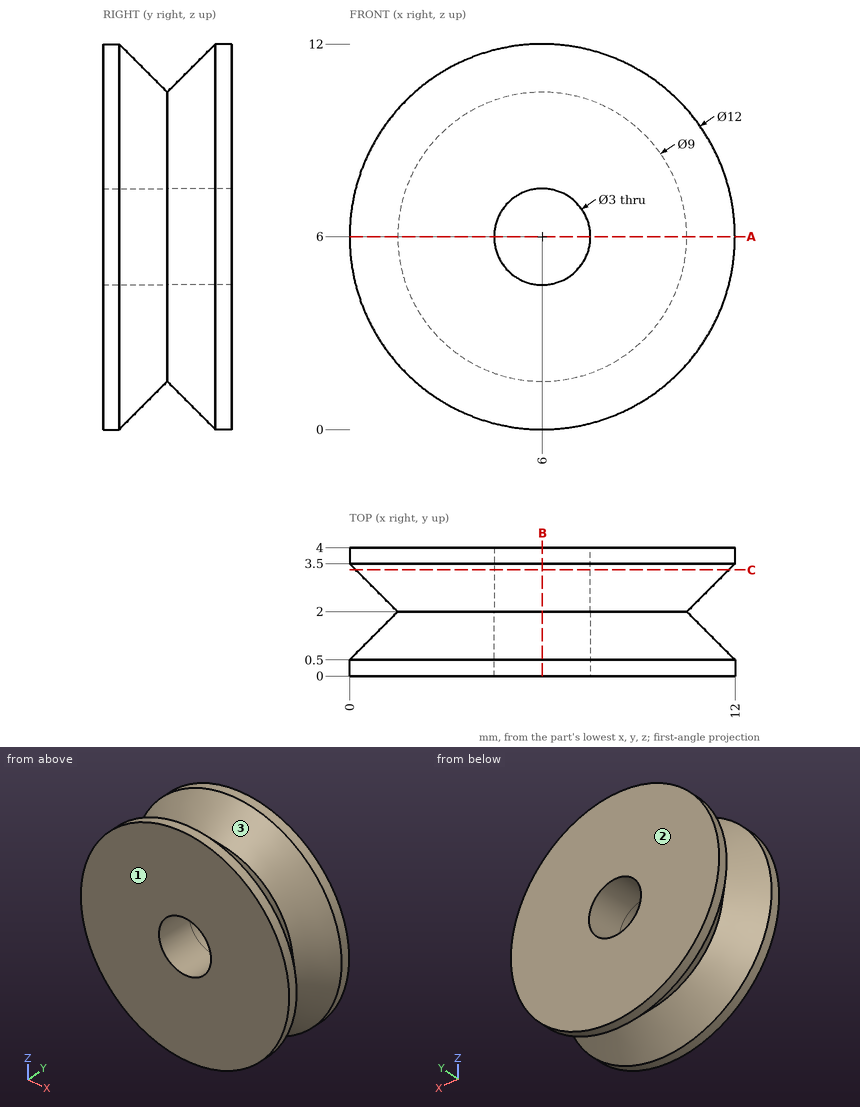
Part print with two shaded views. Sizes in mm from the minimum x, y, z corner. Give positions to 0.01 mm unless a question says otherwise; leave off trailing zeros. Order: outer loops, then holes, each group sorted by start corner. A loop starts at its lowest first (then second) coordinate and runs counter-clockwise, first axis right, second up. Notation, with made-up numbers: M 70.25,55.5 L 89.25,55.5 A14 ccw 89.25,67.5 Z; hole C 14.25,36 d11. An arc over 180 degrees is marked long. Put each result on its own line as item: value.
Item 1: Cut at C-C on y = 3.3. Write the cut outline in (x, z).
Results are:
outline: C 6,6 d11.6; hole C 6,6 d3
Item 2: Cut at A-A on z = 6. Write the cut outline in (x, y).
Results are:
outline: M 0,0 L 4.5,0 L 4.5,4 L 0,4 L 0,3.5 L 1.5,2 L 0,0.5 Z; M 7.5,0 L 12,0 L 12,0.5 L 10.5,2 L 12,3.5 L 12,4 L 7.5,4 Z
Item 3: Pull direction Y, two halves, no side cores. Call the marked faces 1, 2 and 3: +Y half, -Y half, draft (parallel to the pull), parting line (faces both ways), or undercut.
Results are:
face 1: -Y half
face 2: +Y half
face 3: undercut
Item 4: Cut at B-B on x = 6. Write the cut outline in (y, z), then the cut area to 3 significant figures.
Results are:
outline: M 0,0 L 0.5,0 L 2,1.5 L 3.5,0 L 4,0 L 4,4.5 L 0,4.5 Z; M 0,7.5 L 4,7.5 L 4,12 L 3.5,12 L 2,10.5 L 0.5,12 L 0,12 Z
area: 31.5 mm2
Item 5: Wall check: probe 1 along Y at (x, z) = (5, 10.5); probe 2 along Z at (x, y) = (6, 2.7); probe 3 along Z at (x, y) = (6, 3.05). Give the ranges that are in metal, low to high.
Results are:
probe 1: 0 to 1.89, 2.11 to 4
probe 2: 0.8 to 4.5, 7.5 to 11.2
probe 3: 0.45 to 4.5, 7.5 to 11.55
Item 6: Drop flat-ended pins along their axis: pin 1 Ø1 at (x, y) = (2.5, 2) entering from -Z; pin 2 Ø3.5 at (x, z) = (6, 6) entering from +Y; pin 3 Ø2.5 at (x, z) = (6, 6) entering from -Y; pin 4 Ø1.5 at (x, y) = (7, 2.5) entering from -Z. Give the stop position or say it passes through.
Results are:
pin 1: z = 2.29
pin 2: y = 4
pin 3: through
pin 4: z = 0.33
